Check sheet for the modelled part. Datum: model origin and axes. Units: mm. Face numbers are marked on the shaded views. A direction names the side the tool comes from. Round coordinates to 2 decimals unless told otherwise and drop trailing zeros. Write each loop counter-clockwise with the first axis right and the second up, starting at its lowest first coordinate (ties: lowest second). Pieces come first, ordered by that corner, then holes. Notation, with made-up numbers: (9.25, -38) -> (40.25, -38) arc R26 cw to (40.25, -17) -> close; hole circle Ø2 at (-9.5, 83.25). An arc over 180 degrees is marked (long way). Write item = value, one per line.
from build123d import *

# Parameters (mm, degrees)
SKETCH1_W           = 25
SKETCH1_H           = 23.1
SKETCH1_W_2         = 23.1
SKETCH1_H_2         = 25
BOSS_EXTRUDE2_DEPTH = 25.5
SKETCH2_W           = 23.1
SKETCH2_H           = 1.2
CUT_EXTRUDE1_DEPTH  = 25
SKETCH3_W           = 23.1
SKETCH3_H           = 1.2
CUT_EXTRUDE2_DEPTH  = 25
SKETCH4_W           = 23.1
SKETCH4_H           = 1.2
CUT_EXTRUDE3_DEPTH  = 25
SKETCH5_W           = 20
SKETCH5_H           = 20
CUT_EXTRUDE4_DEPTH  = 76.5
SKETCH8_W           = 20
SKETCH8_H           = 20
CUT_EXTRUDE5_DEPTH  = 30
FILLET1_R           = 1


with BuildPart() as part:
    # Sketch1 → Boss-Extrude2 (new body)
    with BuildSketch(Plane(origin=(0, 0, 0), x_dir=(1, 0, 0), z_dir=(0, 1, 0))):
        with Locations((-25.25, 0)):
            Rectangle(SKETCH1_W, SKETCH1_H)
        Polygon((11.55, 12.75), (-11.55, 12.75), (-12.75, 12.75), (-12.75, 11.55), (-12.75, -11.55), (-12.75, -12.75), (12.75, -12.75), (12.75, -11.55), (12.75, 11.55), (12.75, 12.75), align=None)
        with Locations((0, 25.25)):
            Rectangle(SKETCH1_W_2, SKETCH1_H_2)
        with Locations((25.25, 0)):
            Rectangle(SKETCH1_W, SKETCH1_H)
    extrude(amount=BOSS_EXTRUDE2_DEPTH)

    # Sketch2 → Cut-Extrude1 (cut)
    with BuildSketch(Plane(origin=(37.75, 0, 0), x_dir=(0, 0, -1), z_dir=(1, 0, 0))):
        with Locations((0, 24.9)):
            Rectangle(SKETCH2_W, SKETCH2_H)
        with Locations((0, 0.6)):
            Rectangle(SKETCH2_W, SKETCH2_H)
    extrude(amount=-CUT_EXTRUDE1_DEPTH, mode=Mode.SUBTRACT)

    # Sketch3 → Cut-Extrude2 (cut)
    with BuildSketch(Plane.ZY.offset(37.75)):
        with Locations((0, 24.9)):
            Rectangle(SKETCH3_W, SKETCH3_H)
        with Locations((0, 0.6)):
            Rectangle(SKETCH3_W, SKETCH3_H)
    extrude(amount=-CUT_EXTRUDE2_DEPTH, mode=Mode.SUBTRACT)

    # Sketch4 → Cut-Extrude3 (cut)
    with BuildSketch(Plane(origin=(0, 0, -37.75), x_dir=(-1, 0, 0), z_dir=(0, 0, -1))):
        with Locations((0, 24.9)):
            Rectangle(SKETCH4_W, SKETCH4_H)
        with Locations((0, 0.6)):
            Rectangle(SKETCH4_W, SKETCH4_H)
    extrude(amount=-CUT_EXTRUDE3_DEPTH, mode=Mode.SUBTRACT)

    # Sketch5 → Cut-Extrude4 (cut, through all)
    with BuildSketch(Plane(origin=(37.75, 0, 0), x_dir=(0, 0, -1), z_dir=(1, 0, 0))):
        with Locations((0, 12.75)):
            Rectangle(SKETCH5_W, SKETCH5_H)
    extrude(amount=-CUT_EXTRUDE4_DEPTH, mode=Mode.SUBTRACT)

    # Sketch8 → Cut-Extrude5 (cut)
    with BuildSketch(Plane(origin=(0, 0, -37.75), x_dir=(-1, 0, 0), z_dir=(0, 0, -1))):
        with Locations((0, 12.75)):
            Rectangle(SKETCH8_W, SKETCH8_H)
    extrude(amount=-CUT_EXTRUDE5_DEPTH, mode=Mode.SUBTRACT)

    # Fillet1
    fillet1_edges = [part.edges().sort_by_distance(p)[0] for p in [
        (25.25, 1.2, 11.55),
        (37.75, 1.2, 0),
        (-37.75, 12.75, 11.55),
        (-37.75, 12.75, -11.55),
        (-25.25, 24.3, -11.55),
        (-25.25, 24.3, 11.55),
        (-37.75, 24.3, 0),
        (-25.25, 1.2, 11.55),
        (-25.25, 1.2, -11.55),
        (-37.75, 1.2, 0),
        (-11.55, 12.75, -37.75),
        (11.55, 12.75, -37.75),
        (11.55, 24.3, -25.25),
        (-11.55, 24.3, -25.25),
        (0, 24.3, -37.75),
        (-11.55, 1.2, -25.25),
        (11.55, 1.2, -25.25),
        (0, 1.2, -37.75),
        (37.75, 12.75, -11.55),
        (37.75, 12.75, 11.55),
        (25.25, 24.3, 11.55),
        (25.25, 24.3, -11.55),
        (37.75, 24.3, 0),
        (25.25, 1.2, -11.55),
    ]]
    fillet(fillet1_edges, radius=FILLET1_R)


solid = part.part
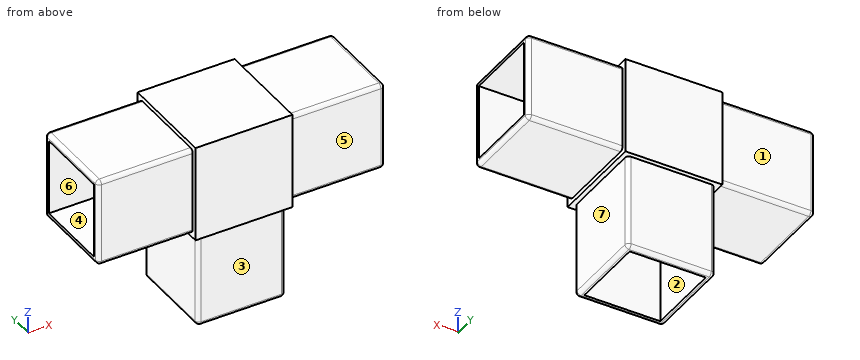
(1) Sectioned sample at D-D on x = -9. Enter the section's corners in (y, z).
Worked answers:
outline = (0, -12.75) -> (1.2, -12.75) -> (1.2, -36.75) arc R1 ccw to (2.2, -37.75) -> (2.75, -37.75) -> (2.75, 10) -> (22.75, 10) -> (22.75, -37.75) -> (23.3, -37.75) arc R1 ccw to (24.3, -36.75) -> (24.3, -12.75) -> (25.5, -12.75) -> (25.5, 12.75) -> (0, 12.75) -> close
(2) Sectioned sample at A-A on y = 12.75. Count the separate pieces of the cut face and the enclosed holes in it, then the cut area to 3 significant figures.
Worked answers:
separate_pieces = 3
enclosed_holes = 0
area = 316 mm²
(3) Release check for a two-part mould opening along X. For the marked faces 5, 6 and 7 record: pulls with the +X half, pulls with the -X half, needs draft (parallel to the pull), parting line crosses it, or undercut.
Worked answers:
face_5 = needs draft
face_6 = undercut
face_7 = pulls with the +X half
(4) Access from +Z, -Z, +X, -X, +Y, -Y to the whole of each face (thin tool, end or side, straight path). Record for the marked faces 1, 2, 3 and 4.
Worked answers:
face_1 = +Z, -Z, -X, +Y
face_2 = -Z
face_3 = -Z, +X, -X, -Y
face_4 = +X, -X
(5) Go/stop test with flat-tipped pins: P1, Ø1, axis at x = -19.5, z = -6.5, coming from the -Y side; P2, Ø10.5, axis at y = 10.5, z = -20.5, coming from the +X side; P3, Ø6, axis at y = 8, z = -32, coming from the -X side; P4, Ø7.5, axis at y = 15, z = -5.5, coming from the -X side. Record where each tip stops, or that it passes through.
Worked answers:
P1 = 1.2
P2 = 11.55
P3 = -11.55
P4 = through
(6) Sectioned sample at B-B on z = 7.5. Enter the section's corners in (x, y), then the cut area to 3 significant figures.
Worked answers:
outline = (-37.75, 2.2) arc R1 ccw to (-36.75, 1.2) -> (-12.75, 1.2) -> (-12.75, 0) -> (12.75, 0) -> (12.75, 1.2) -> (36.75, 1.2) arc R1 ccw to (37.75, 2.2) -> (37.75, 2.75) -> (-37.75, 2.75) -> close; (-37.75, 22.75) -> (37.75, 22.75) -> (37.75, 23.3) arc R1 ccw to (36.75, 24.3) -> (12.75, 24.3) -> (12.75, 25.5) -> (-12.75, 25.5) -> (-12.75, 24.3) -> (-36.75, 24.3) arc R1 ccw to (-37.75, 23.3) -> close
area = 294 mm²
(7) Sectioned sample at C-C on x = -18.5. Enter the section's corners in (y, z).
Worked answers:
outline = (1.2, -10.55) arc R1 ccw to (2.2, -11.55) -> (23.3, -11.55) arc R1 ccw to (24.3, -10.55) -> (24.3, 10.55) arc R1 ccw to (23.3, 11.55) -> (2.2, 11.55) arc R1 ccw to (1.2, 10.55) -> close; hole (2.75, -10) -> (22.75, -10) -> (22.75, 10) -> (2.75, 10) -> close
(8) Material ranges on L1, parallel to Z at x = 17, y = 9.25; L2, parallel to Y at x = -8, z = -14.5, recorded low to high. Write a range as [from, to].
Worked answers:
L1 = [-11.55, -10], [10, 11.55]
L2 = [1.2, 2.75], [22.75, 24.3]
